Model file for the job. Use its own axes, mm. A direction names the side the tool comes from. Round coordinates to 2 decimals unless told otherwise and drop trailing zeros. Order: outer loops, then holes, each group sorted by start corner. A loop starts at its lowest first (then second) coordinate and runs counter-clockwise, first axis right, second up. Notation, with made-up numbers: (10, 55.5) - (32, 55.5) arc R31 ccw to (32, 90.5) - close; hole circle Ø7 at (77.25, -9.5). An arc over 180 degrees is marked (long way). Put each result on its own line as item: value. Start each with the question number.
Item 1: Probe probe 1 along Z at (x, y) = (2.5, 40); probe 2 along X at (y, z) = (41, 24); probe 3 along X at (y, z) = (16.5, -26.5). List the from-to ranges inside material, lowest first.
Item 2: Mould opens along Z. For faces 5 (the face through (-17.575, 1.479, -45.8)), 6 (the face through (-39, 3, -27)), 7 (the face through (4.19, 93.99, -3.52)) say: pulls with the +Z half, pulls with the -Z half, needs draft (parallel to the pull), parting line crosses it, or undercut.
Item 3: Pin check, flat tips, straight feed: pin 1 Ø5.5 at (x, z) = (-0.5, -2.5) entering from -Y; pin 2 Ø3.5 at (x, y) = (-48.5, 2) entering from +Z; pin 3 Ø4 at (x, y) = (-23.5, 58) entering from +Z; pin 4 Ø5 at (x, z) = (-2.44, -2.51) entering from +Y. Stop position of each tip, or through.
Item 4: Saw through at B-B on y = 38.5. List the corners of the cut face in (x, z), plus the area to 3 significant figures.
Item 5: Saw through at A-A on y = 22.5. List the corners of the cut face in (x, z), plus the area to 3 significant figures.
Item 6: Which spindle directions (+Z, -Z, +X, -X, +Y, -Y) get a long thin tool onto all of the face, cutting with end or side? Do faces 1 (the face through (-3.66, 93.99, -0.92)), 2 (the face through (29, 25, -32)), 3 (the face through (37.944, 12.325, 24.192)), 4 (the face through (-49, 1, 0)). Say none if no direction does.
```python
from build123d import *

# Parameters (mm, degrees)
SKETCH_1_R          = 45
SKETCH_1_R_2        = 43.5
EXTRUDE_1_DEPTH     = 25
EXTRUDE_2_DEPTH     = 3
SKETCH_6_R          = 2
CUT_EXTRUDE_1_DEPTH = 3


# Read off the part's stored shape, not the designer's step: 抽壳9
with BuildPart() as part:
    # 草图1 → 凸台-拉伸1 (new body)
    with BuildSketch(Plane(origin=(0, 0, 0), x_dir=(1, 0, 0), z_dir=(0, 1, 0))):
        with Locations(Location((0, 0, 0), (0, 0, 270))):
            Circle(SKETCH_1_R)
        with Locations(Location((0, 0, 0), (0, 0, 270))):
            Circle(SKETCH_1_R_2, mode=Mode.SUBTRACT)
    extrude(amount=EXTRUDE_1_DEPTH)

    # 草图2 → 凸台-拉伸2 (add)
    with BuildSketch(Plane(origin=(0, 0, 0), x_dir=(1, 0, 0), z_dir=(0, 1, 0))):
        with BuildLine():
            Line((-45, 0), (-53, 0))
            ThreePointArc((-53, 0), (-45.144679687, 31.028280094), (-18.991709994, 49.480445253))
            Line((-18.991709994, 49.480445253), (-16.117646372, 42.014538858))
            ThreePointArc((-16.117646372, 42.014538858), (-37.082975115, 25.492213647), (-45, 0))
        make_face()
    extrude(amount=EXTRUDE_2_DEPTH)

    # 草图5 → 旋转3 (revolve)
    with BuildSketch(Plane.XY, mode=Mode.PRIVATE) as revolve_3_sk:
        Polygon((-45, 25), (0, 25), (0, 95), (-10, 95), align=None)
    revolve(revolve_3_sk.sketch.rotate(Axis((0, 25, 0), (0, 1, 0)), 270), axis=Axis((0, 25, 0), (0, 1, 0)))

    # 抽壳9 outline → 抽壳9 (revolve, cut)
    with BuildSketch(Plane.XY):
        Polygon((42.763932023, 25), (8.763932023, 93), (0, 93), (0, 25), align=None)
    revolve(axis=Axis((0, 0, 0), (0, 1, 0)), mode=Mode.SUBTRACT)

    # 草图6 → 切除-拉伸1 (cut)
    with BuildSketch(Plane.XZ.offset(-93)):
        with Locations(Location((-2.574448684, 2.371120826, 0), (0, 0, 270))):
            Circle(SKETCH_6_R)
        with Locations(Location((2.6320911, 2.306966935, 0), (0, 0, 270))):
            Circle(SKETCH_6_R)
        with Locations(Location((-2.443496184, -2.505858416, 0), (0, 0, 270))):
            Circle(SKETCH_6_R)
        with Locations(Location((2.504843697, -2.444536368, 0), (0, 0, 270))):
            Circle(SKETCH_6_R)
    extrude(amount=-CUT_EXTRUDE_1_DEPTH, mode=Mode.SUBTRACT)


solid = part.part
```
Results found:
1. probe 1: z = -37.42 to -35.18, 35.18 to 37.42
1. probe 2: x = -28.16 to -25.15, 25.15 to 28.16
1. probe 3: x = -36.37 to -34.5, 34.5 to 36.37
2. face 5: pulls with the -Z half
2. face 6: needs draft
2. face 7: undercut
3. pin 1: stops at y = 93
3. pin 2: stops at z = 0
3. pin 3: stops at z = 19.17
3. pin 4: stops at y = 95
4. outline: circle Ø76.5 at (0, 0); hole circle Ø72.03 at (0, 0)
4. area: 522 mm²
5. outline: circle Ø90 at (0, 0); hole circle Ø87 at (0, 0)
5. area: 417 mm²
6. face 1: +Y, -Y
6. face 2: -Y
6. face 3: +Y
6. face 4: +Z, -X, +Y, -Y
